```python
from build123d import *

# Parameters (mm, degrees)
F0_W     = 50.8
F0_H     = 48.42591
F1_DEPTH = 50.8
F2_W     = 51.555392
F2_H     = 49.770784
F3_DEPTH = 0.254


with BuildPart() as f1:
    # F0 (on Top) → F1 (new body)
    with BuildSketch(Plane.XY):
        with BuildLine():
            ThreePointArc((31.75, 22.785854), (29.890128, 27.275982), (25.4, 29.135854))
            Line((25.4, 29.135854), (-25.4, 29.135854))
            ThreePointArc((-25.4, 29.135854), (-29.890128, 27.275982), (-31.75, 22.785854))
            Line((-31.75, 22.785854), (-31.75, -22.785854))
            ThreePointArc((-31.75, -22.785854), (-29.890128, -27.275982), (-25.4, -29.135854))
            Line((-25.4, -29.135854), (25.4, -29.135854))
            ThreePointArc((25.4, -29.135854), (29.890128, -27.275982), (31.75, -22.785854))
            Line((31.75, -22.785854), (31.75, 22.785854))
        make_face()
        Rectangle(F0_W, F0_H, mode=Mode.SUBTRACT)
    extrude(amount=F1_DEPTH)

    # F2 (on Top) → F3 (join)
    with BuildSketch(Plane.XY):
        Rectangle(F2_W, F2_H)
    extrude(amount=F3_DEPTH)


solid = f1.part
```
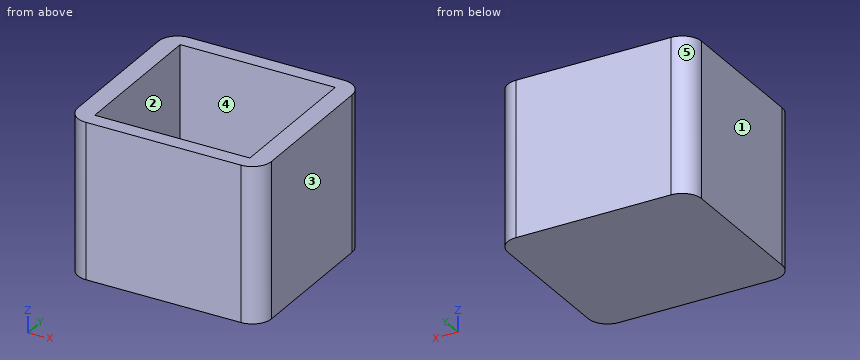
Check sheet for the modelled part. Datum: model origin and axes. Units: mm. Face numbers are marked on the shaded views. A direction names the side the tool comes from. Coordinates: 2 decimals unless noted, no trailing zeros. Order: outer loops, then holes, each group sorted by start corner. A loop starts at its lowest first (then second) coordinate and runs counter-clockwise, first axis right, second up. Notation, with made-up numbers: (-4.5, 24) -> (20.5, 24) arc R25 ccw to (20.5, 49) -> close; hole circle Ø5 at (42, 37). An arc over 180 degrees is marked (long way). Write each question's results on one line, items separated by ' | '. Start each with the question number.
1) Depth check by flat-ended pin: pin 1 (14.5 mm diameter, centred on x = -8.5, y = 8.5, fed in from +Z). Enter the tip coordinate at first touch or a pass-through.
2) Set-up check for the marked faces 4 and 5: record each of +Z, -Z, +X, -X, +Y, -Y from which the full face is reachable in a straight line by a thin tool's end or side.
3) Section check C-C (x = 10.5). Enter the section's corners in (y, z), and give its area (3 significant figures).
4) Draft check along X on the marked faces 1, 2 and 3. Enter one of: pulls with the +X half, pulls with the -X half, needs draft (parallel to the pull), parting line crosses it, or undercut.
5) Section check A-A (z = 23). Enter the section's corners in (x, y), and give its area (3 significant figures).
6) Section check B-B (y = 7). Enter the section's corners in (x, z).
7) Material ranges on line 1 along Y through (x, z) = (-19, 32); line 2 along X through (y, z) = (-15, 28.5); line 3 along Z through (x, y) = (13, -13), recorded low to high.
Checked values:
1) pin 1: z = 0.25
2) face 4: +Z | face 5: +Z, -Z, -X, +Y
3) outline: (-29.14, 0) -> (29.14, 0) -> (29.14, 50.8) -> (24.21, 50.8) -> (24.21, 0.25) -> (-24.21, 0.25) -> (-24.21, 50.8) -> (-29.14, 50.8) -> close | area: 512 mm²
4) face 1: pulls with the -X half | face 2: undercut | face 3: pulls with the +X half
5) outline: (-31.75, -22.79) arc R6.35 ccw to (-25.4, -29.14) -> (25.4, -29.14) arc R6.35 ccw to (31.75, -22.79) -> (31.75, 22.79) arc R6.35 ccw to (25.4, 29.14) -> (-25.4, 29.14) arc R6.35 ccw to (-31.75, 22.79) -> close; hole (-25.4, -24.21) -> (25.4, -24.21) -> (25.4, 24.21) -> (-25.4, 24.21) -> close | area: 1,210 mm²
6) outline: (-31.75, 0) -> (31.75, 0) -> (31.75, 50.8) -> (25.4, 50.8) -> (25.4, 0.25) -> (-25.4, 0.25) -> (-25.4, 50.8) -> (-31.75, 50.8) -> close
7) line 1: -29.14 to -24.21, 24.21 to 29.14 | line 2: -31.75 to -25.4, 25.4 to 31.75 | line 3: 0 to 0.25
